from build123d import *

# Parameters (mm, degrees)
SKETCH2_W          = 0.25
SKETCH2_H          = 1.125
SKETCH2_W_2        = 1.125
SKETCH2_H_2        = 0.25
CUT_EXTRUDE1_DEPTH = 0.5


with BuildPart() as part:
    # Sketch1 → Revolve1 (revolve)
    with BuildSketch(Plane.XY, mode=Mode.PRIVATE) as revolve1_sk:
        Polygon((0, 0), (1.6, 0), (1.6, -1), (0.9, -1), (0.9, -33.5), (0, -33.5), align=None)
    revolve(revolve1_sk.sketch.rotate(Axis((0, -33.5, 0), (0, 1, 0)), 90), axis=Axis((0, -33.5, 0), (0, 1, 0)))

    # Sketch2 → Cut-Extrude1 (cut)
    with BuildSketch(Plane(origin=(0, 0, 0), x_dir=(1, 0, 0), z_dir=(0, 1, 0))):
        with Locations((0, -0.6875)):
            Rectangle(SKETCH2_W, SKETCH2_H)
        with Locations((-0.6875, 0)):
            Rectangle(SKETCH2_W_2, SKETCH2_H_2)
        with Locations((0, 0.6875)):
            Rectangle(SKETCH2_W, SKETCH2_H)
        with Locations((0.6875, 0)):
            Rectangle(SKETCH2_W_2, SKETCH2_H_2)
        Rectangle(SKETCH2_W, SKETCH2_H_2)
    extrude(amount=-CUT_EXTRUDE1_DEPTH, mode=Mode.SUBTRACT)


solid = part.part
Geometry check sheet. Reference: the model listing, model coordinates, mm. Round coordinates to 2 decimals unless told otherwise and drop trailing zeros. Write each loop counter-clockwise with the first axis right and the second up, starting at its lowest first coordinate (ties: lowest second). Pieces come first, ordered by that corner, then holes.
Item 1: Material ranges on line 1 along Y through (x, z) = (-0.95, -0.9); line 2 along X through (y, z) = (-4, 0.05), recorded low to high.
Determined:
line 1: y = -1 to 0
line 2: x = -0.9 to 0.9
Item 2: Section check B-B (y = -11.5). Record the boundary of the cut face in (x, z), plus the area to 3 significant figures.
Determined:
outline: circle Ø1.8 at (0, 0)
area: 2.54 mm2
Item 3: Mould release check, pull along Y, two halves, no side actions. Record for faces 1 (the face through (1, -1, -1)), 2 (the face through (-0.27, -17.48, -0.86)), 3 (the face through (0.3, 0, 0.3)): +Y half, -Y half, draft (parallel to the pull), parting line (faces both ways), or undercut.
Determined:
face 1: -Y half
face 2: draft
face 3: +Y half
Item 4: Section check A-A (x = -0.6). Record the boundary of the cut face in (y, z) (3 decimals).
Determined:
outline: (-33.5, -0.671) - (-1, -0.671) - (-1, -1.483) - (0, -1.483) - (0, -0.125) - (-0.5, -0.125) - (-0.5, 0.125) - (0, 0.125) - (0, 1.483) - (-1, 1.483) - (-1, 0.671) - (-33.5, 0.671) - close
Item 5: Go/stop test with a flat-tipped pin: pin 1 Ø0.6 at (y, z) = (0, -0.5) entering from -X. Record where the tip stops, or that it passes through.
Determined:
pin 1: stops at x = -1.59
